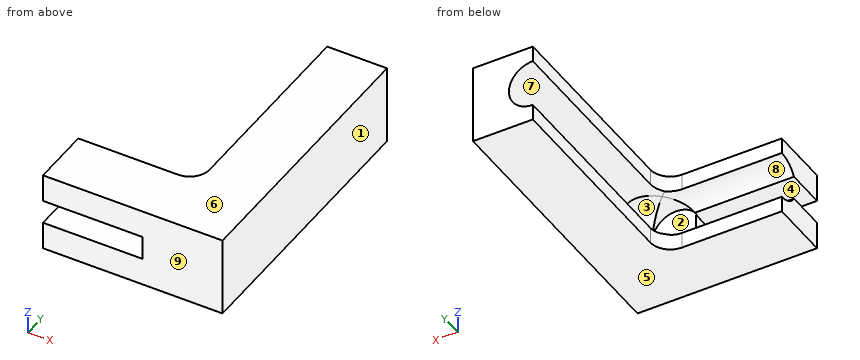
from build123d import *

# Parameters (mm, degrees)
F1_DEPTH = 20
F2_R     = 6
F3_DEPTH = 40
F4_R     = 6
F5_DEPTH = 61
F6_W     = 25
F6_H     = 6
F7_DEPTH = 25


with BuildPart() as f1:
    # F0 (on Top) → F1 (new body)
    with BuildSketch(Plane.XY):
        with BuildLine():
            Line((22.5, 35), (7.5, 35))
            Line((7.5, 35), (7.5, -15))
            ThreePointArc((7.5, -15), (6.035534, -18.535534), (2.5, -20))
            Line((2.5, -20), (-22.5, -20))
            Line((-22.5, -20), (-22.5, -35))
            Line((-22.5, -35), (22.5, -35))
            Line((22.5, -35), (22.5, 35))
        make_face()
    extrude(amount=F1_DEPTH)

    # F2 (on face) → F3 (cut)
    with BuildSketch(Plane(origin=(-22.5, 0, 0), x_dir=(0, -1, 0), z_dir=(-1, 0, 0))):
        with Locations((20, 10)):
            Circle(F2_R)
    extrude(amount=-F3_DEPTH, mode=Mode.SUBTRACT)

    # F4 (on face) → F5 (cut)
    with BuildSketch(Plane(origin=(0, 35, 0), x_dir=(-1, 0, 0), z_dir=(0, 1, 0))):
        with Locations((-7.5, 10)):
            Circle(F4_R)
    extrude(amount=-F5_DEPTH, mode=Mode.SUBTRACT)

    # F6 (on face) → F7 (cut)
    with BuildSketch(Plane.XZ.offset(35)):
        with Locations((-10, 10)):
            Rectangle(F6_W, F6_H)
    extrude(amount=-F7_DEPTH, mode=Mode.SUBTRACT)


solid = f1.part
Geometry check sheet. Reference: the model listing, model coordinates, mm. Face numbers are marked on the shaded views. A direction names the side the tool comes from. Give positions to 0.01 mm unless a question says otherwise; leave off trailing zeros. Loops run counter-clockwise (first coordinate to the right, second up) from the corner with the lowest first, then second, coordinate; pieces in that order, holes last. Notation, with made-up numbers: M -2.75,-18 L 46.25,-18 A29 cw 46.25,8 Z; hole C -33,-22.75 d3. An arc over 180 degrees is marked long. Answer as a JSON object with one key per item and string values. Group by question number.
Item 1: Sectioned sample at C-C on z = 10.75. Record the boundary of the cut face in (x, y), plus the area to 3 significant figures.
Item 2: Sectioned sample at D-D on y = 30. Record the boundary of the cut face in (x, z), plus the area to 3 significant figures.
Item 3: Sectioned sample at A-A on x = -19. Record the boundary of the cut face in (y, z), plus the area to 3 significant figures.
Item 4: Mould release check, pull along Z, two halves, no side actions. Record for the marked faces 6, 7, 8 and 9: pulls with the +Z half, pulls with the -Z half, needs draft (parallel to the pull), parting line crosses it, or undercut.
Item 5: Material ranges on L1, parallel to Z at x = -15, y = -21.5; L2, parallel to Z at x = -10, y = -28.5; L3, parallel to X at y = -9.5, z = 1.5, recorded low to high.
Item 6: Access from +Z, -Z, +X, -X, +Y, -Y to the whole of each face (thin tool, end or side, straight path). Record for the marked faces 1, 2, 3, 4 and 5.
Item 7: Gauge pin test, flat ends, axial feed: pin 1 (2 mm diameter, centred on x = -6.5, z = 17, fed in from +Y); pin 2 (6 mm diameter, centred on x = 2.5, z = 8.5, fed in from +Y); pin 3 (2 mm diameter, centred on y = -2, z = 19, fed in from -X). Record the tip position at first contact, or that the pin passes through.
Item 8: Sectioned sample at B-B on y = -30. Record the boundary of the cut face in (x, z), plus the area to 3 significant figures.
Findings below:
{
 "1": {"outline": "M 2.5,-35 L 22.5,-35 L 22.5,35 L 13.45,35 L 13.45,-14.05 L 17.5,-14.05 L 17.5,-25.95 L 13.45,-25.95 L 13.45,-26 L 2.5,-26 Z", "area": "684 mm2"},
 "2": {"outline": "M 7.5,0 L 22.5,0 L 22.5,20 L 7.5,20 L 7.5,16 A6 cw 7.5,4 Z", "area": "243 mm2"},
 "3": {"outline": "M -35,0 L -20,0 L -20,4 A6 cw -25.2,7 L -35,7 Z; M -35,13 L -25.2,13 A6 cw -20,16 L -20,20 L -35,20 Z", "area": "188 mm2"},
 "4": {"face 6": "pulls with the +Z half", "face 7": "undercut", "face 8": "undercut", "face 9": "needs draft"},
 "5": {"L1": "0 to 4.19, 15.81 to 20", "L2": "0 to 7, 13 to 20", "L3": "7.5 to 22.5"},
 "6": {"face 1": "+Z, -Z, +X, +Y, -Y", "face 2": "+Y", "face 3": "-X", "face 4": "-X, +Y, -Y", "face 5": "-Z, +X, -X, +Y, -Y"},
 "7": {"pin 1": "y = -20", "pin 2": "y = -23.97", "pin 3": "x = 7.5"},
 "8": {"outline": "M -22.5,0 L 22.5,0 L 22.5,20 L -22.5,20 L -22.5,13 L 2.5,13 L 2.5,7 L -22.5,7 Z", "area": "750 mm2"}
}
